The model under review builds one solid part; all positions refer to its coordinate system, in mm. A direction names the side the tool comes from. Coordinates: 2 decimals unless noted, no trailing zeros. Order: outer loops, then holes, each group sorted by start corner. A loop starts at its lowest first (then second) coordinate and runs counter-clockwise, first axis right, second up. Notation, with made-up numbers: (0, 66.25) -> (41, 66.25) arc R9 cw to (41, 72.25) -> close; hole circle Ø10 at (4.5, -29). An arc over 180 degrees is marked (long way). Put each result on its own line as item: value.
from build123d import *

# Parameters (mm, degrees)
F0_W     = 88.9
F0_H     = 88.9
F1_DEPTH = 1219.2
F2_W     = 50.8
F2_H     = 38.1
F3_DEPTH = 101.6
F4_W     = 88.9
F4_H     = 88.9
F4_W_2   = 44.45
F4_H_2   = 44.45
F5_DEPTH = 50.8


with BuildPart() as f1:
    # F0 (on Front) → F1 (new body)
    with BuildSketch(Plane.XZ):
        with Locations((44.45, 44.45)):
            Rectangle(F0_W, F0_H)
    extrude(amount=F1_DEPTH)

    # F2 (on face) → F3 (cut)
    with BuildSketch(Plane.YZ.offset(88.9)):
        with Locations((-1193.8, 44.45)):
            Rectangle(F2_W, F2_H)
    extrude(amount=-F3_DEPTH, mode=Mode.SUBTRACT)

    # F4 (on face) → F5 (cut)
    with BuildSketch(Plane(origin=(0, 0, 0), x_dir=(-1, 0, 0), z_dir=(0, 1, 0))):
        with Locations((-44.45, 44.45)):
            Rectangle(F4_W, F4_H)
        with Locations((-44.45, 44.45)):
            Rectangle(F4_W_2, F4_H_2, mode=Mode.SUBTRACT)
    extrude(amount=-F5_DEPTH, mode=Mode.SUBTRACT)


solid = f1.part
Item 1: For line 1 (Y direction, x = 32, z = 78.5); line 2 (Y direction, x = 60, z = 34.5), list the stretches that pass through material, from the lowest coordinate up. Write a range as from..to.
Answers below:
line 1: -1219.2..-50.8
line 2: -1168.4..0
Item 2: For pin 1 Ø19 at (x, z) = (55, 48) entering from -Y, flat-tipped, find the tip position at first contact; note if it passes through.
Answers below:
pin 1: y = -1168.4
Item 3: Mouldability with a two-part tool opening along Z and no side actions: class faces 6 (the flat face through (44, 0, 45)), 7 (the flat face through (45, -1194, 63.5)), 8 (the flat face through (44, -627, 88.9)) as +Z half, -Z half, draft (parallel to the pull), parting line (faces both ways), or undercut.
Answers below:
face 6: draft
face 7: undercut
face 8: +Z half
Item 4: For faces 1 (the flat face through (45, -25, 66.675)), 2 (the flat face through (45, -1194, 25.4)), 3 (the flat face through (22.225, -25, 44)), 4 (the flat face through (45, -25, 22.225)), 5 (the flat face through (66.675, -25, 44)), list the 3-axis set-ups (+Z, -Z, +X, -X, +Y, -Y) from which the entire face can be reached by the end or side of a thin tool; tool diameter is ignored.
Answers below:
face 1: +Z, +X, -X, +Y
face 2: +X, -X, -Y
face 3: +Z, -Z, -X, +Y
face 4: -Z, +X, -X, +Y
face 5: +Z, -Z, +X, +Y
Item 5: Consider section B-B on z = 51. Write out the cut boundary in (x, y) (3 decimals), and give its area (3 significant figures).
Answers below:
outline: (0, -1168.4) -> (88.9, -1168.4) -> (88.9, -50.8) -> (66.675, -50.8) -> (66.675, 0) -> (22.225, 0) -> (22.225, -50.8) -> (0, -50.8) -> close
area: 102,000 mm^2
Item 6: Consider section A-A on x = 77.5. Write out the cut boundary in (y, z), and give its area (3 significant figures).
Answers below:
outline: (-1219.2, 0) -> (-50.8, 0) -> (-50.8, 88.9) -> (-1219.2, 88.9) -> (-1219.2, 63.5) -> (-1168.4, 63.5) -> (-1168.4, 25.4) -> (-1219.2, 25.4) -> close
area: 102,000 mm^2
